from build123d import *

# Parameters (mm, degrees)
F2_R     = 4.55
F3_DEPTH = 25.4
F4_DEPTH = 25.4
F5_SIZE  = 3
F6_R     = 10
F7_SIZE  = 5.08


with BuildPart() as f1:
    # F0 (on Front) → F1 (revolve)
    with BuildSketch(Plane.XZ):
        Polygon((-50.647253, 53.75), (-50.647253, 43.45), (-43.517253, 41.81), (-35.187253, 41.81), (-35.187253, 32.5), (-26.757253, 32.5), (-5.610722, 53.779667), (-0.672578, 58.748901), (7.293111, 50.83305), (-13.787253, 33.353894), (-18.744158, 28.883305), (-29.087253, 19.554958), (-29.087253, 15), (-13.787253, 17.013894), (-13.787253, 20.423894), (13.142747, 20.423894), (13.142747, 28.333894), (-5.157253, 28.333894), (-5.157253, 32.843894), (17.578436, 48.34), (19.998436, 48.34), (19.998436, 54.86), (13.998436, 54.86), (9.798436, 53.354149), (1.832747, 61.27), (29.752747, 61.27), (29.752747, 53.75), (44.492747, 53.75), (44.492747, 68.15), (-6.657253, 68.15), (-22.807253, 52.05), (-34.107253, 52.05), (-34.107253, 68.15), (-45.647253, 68.15), (-45.647253, 53.75), align=None)
    revolve(axis=Axis((-3.077253, 0, 0), (1, 0, 0)))

    # F2 (on face) → F3 (cut)
    with BuildSketch(Plane(origin=(-45.647253, 0, 0), x_dir=(0, -1, 0), z_dir=(-1, 0, 0))):
        with Locations((0, 60.91)):
            Circle(F2_R)
    extrude(amount=-F3_DEPTH, mode=Mode.SUBTRACT)

    # F2 (on face) → F4 (cut)
    with BuildSketch(Plane(origin=(-45.647253, 0, 0), x_dir=(0, -1, 0), z_dir=(-1, 0, 0))):
        with Locations((0, 60.91)):
            Circle(F2_R)
        with Locations((-43.069874, 43.069874)):
            Circle(F2_R)
        with Locations((-60.91, 0)):
            Circle(F2_R)
        with Locations((-43.069874, -43.069874)):
            Circle(F2_R)
        with Locations((0, -60.91)):
            Circle(F2_R)
        with Locations((43.069874, -43.069874)):
            Circle(F2_R)
        with Locations((60.91, 0)):
            Circle(F2_R)
        with Locations((43.069874, 43.069874)):
            Circle(F2_R)
    extrude(amount=-F4_DEPTH, mode=Mode.SUBTRACT)

    # F5
    f5_edges = [f1.edges().sort_by_distance(p)[0] for p in [
        (44.492747, 0, -53.75),
    ]]
    chamfer(f5_edges, length=F5_SIZE)

    # F6
    f6_edges = [f1.edges().sort_by_distance(p)[0] for p in [
        (-26.757253, 0, -32.5),
    ]]
    fillet(f6_edges, radius=F6_R)

    # F7
    f7_edges = [f1.edges().sort_by_distance(p)[0] for p in [
        (29.752747, 0, -53.75),
    ]]
    chamfer(f7_edges, length=F7_SIZE)


solid = f1.part
The model under review builds one solid part; all positions refer to its coordinate system, in mm. A direction names the side the tool comes from. Give positions to 0.01 mm unless a question says otherwise; leave off trailing zeros. Order: outer loops, then holes, each group sorted by start corner. A loop starts at its lowest first (then second) coordinate and runs counter-clockwise, first axis right, second up. Notation, with made-up numbers: M 73.5,-14.75 L 97.5,-14.75 A38 ccw 97.5,24.25 Z; hole C 22.25,37.25 d7. An arc over 180 degrees is marked long. Answer in a Markdown table with one row per item. Add a question column.
1. To check wall thickness, follow line 1 along Z through (x, y) = (-38, 0); line 2 along Z through (x, y) = (39.5, 0); line 3 along Y through (x, z) = (9, 0). State the ranges of each line that lie inside material, in increasing order.
2. Add section B-B on x = -20.5. State the section outline as (y, z) points, plus the area to 3 significant figures.
3. For pin 1 Ø1.5 at (x, z) = (34.5, -8.5) entering from -Y; pin 2 Ø6 at (y, z) = (46, 37) entering from -X; pin 3 Ø8 at (x, z) = (28.5, -32.5) entering from -Y, all flat-tipped, find the tip position at first contact; note any pin that passes through.
4. Add section A-A on x = -38.5. Count the separate pieces of the cut face and the enclosed holes in it, plus the area to 3 significant figures.
5. Machinability: for faces 1 (the cylindrical face through (-39.96, 66.53, -14.77)), 2 (the flat face through (-13.787, -17, 5)), 3 (the flat face through (-29.087, 11.5, 10)), 4 (the cylindrical face through (16.956, -16.478, 52.327)), which of the approach directions +Z, -Z, +X, -X, +Y, -Y give a long, thin tool a straight path to every point of the face, cutting with its end or side? Answer none if there is none.
6. Mouldability with a two-part tool opening along X and no side actions: class faces 5 (the flat face through (29.753, -55, -23)), 6 (the conical face through (-43.863, -12.583, 39.955)), 7 (the flat face through (13.143, 19, -8)), 8 (the cylindrical face through (-0.134, -6.135, 19.481)) as released by +X, released by -X, zero draft, split by the parting line, or undercut.
The answers:
| question | item | result |
|---|---|---|
| 1 | line 1 | -68.15 to -65.46, -56.36 to -41.81, 41.81 to 56.36, 65.46 to 68.15 |
| 1 | line 2 | -68.15 to -53.75, 53.75 to 68.15 |
| 1 | line 3 | -68.15 to -61.27, -54.15 to -42.49, -28.33 to -20.42, 20.42 to 28.33, 42.49 to 54.15, 61.27 to 68.15 |
| 2 | outline | C 0,0 d108.7; C 0,0 d54.6; hole C 0,0 d77.59; hole C 0,0 d32.26 |
| 2 | area | 6,080 mm2 |
| 3 | pin 1 | y = -67.71 |
| 3 | pin 2 | x = -45.65 |
| 3 | pin 3 | y = -61.9 |
| 4 | separate pieces | 1 |
| 4 | enclosed holes | 9 |
| 4 | area | 8,580 mm2 |
| 5 | face 1 | +X, -X |
| 5 | face 2 | +X |
| 5 | face 3 | -X |
| 5 | face 4 | none |
| 6 | face 5 | undercut |
| 6 | face 6 | released by -X |
| 6 | face 7 | released by +X |
| 6 | face 8 | zero draft |
